Here's how the part is built. I have some questions about the finished solid (model axes, mm). Face numbers are marked on the shaded views. A direction names the side the tool comes from. Give positions to 0.01 mm unless a question says otherwise; leave off trailing zeros. Write each loop counter-clockwise with the first axis right and the second up, starting at its lowest first coordinate (ties: lowest second). Pieces come first, ordered by that corner, then holes. Notation, with made-up numbers: (65.25, -26.5) -> (94.25, -26.5) arc R35 ccw to (94.25, 6.5) -> close; hole circle Ø1 at (46, 18.5). An arc over 180 degrees is marked (long way). Use one line per item in the form item = value.
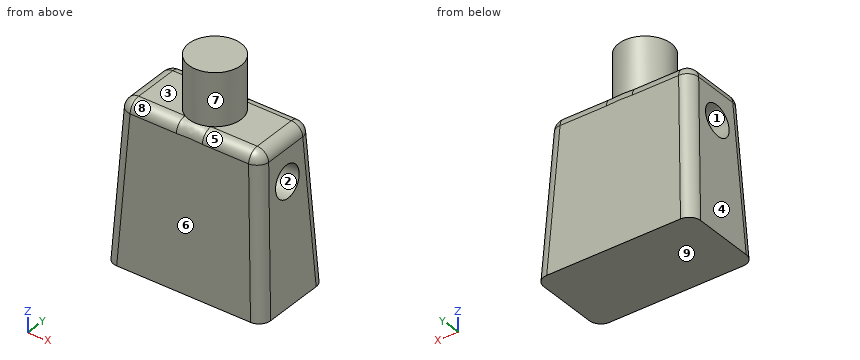
```python
from build123d import *

# Parameters (mm, degrees)
F0_W     = 15
F0_H     = 8
F1_DEPTH = 15
F1_TAPER = 3
F2_R     = 2.5
F3_DEPTH = 5
F4_R     = 1.1
F5_R     = 1.5
F6_DEPTH = 3
F7_R     = 1.5
F8_DEPTH = 3


with BuildPart() as f1:
    # F0 (on Top) → F1 (new body)
    with BuildSketch(Plane.XY):
        Rectangle(F0_W, F0_H)
    extrude(amount=F1_DEPTH, taper=F1_TAPER)

    # F2 (on face) → F3 (join)
    with BuildSketch(Plane.XY.offset(15)):
        Circle(F2_R)
    extrude(amount=F3_DEPTH)

    # F4
    f4_edges = [f1.edges().sort_by_distance(p)[0] for p in [
        (7.106942, 3.606942, 7.5),
        (-7.106942, 3.606942, 7.5),
        (0, 3.213883, 15),
        (-6.713883, 0, 15),
        (6.713883, 0, 15),
        (0, -3.213883, 15),
        (7.106942, -3.606942, 7.5),
        (-7.106942, -3.606942, 7.5),
    ]]
    fillet(f4_edges, radius=F4_R)

    # F5 (on face) → F6 (cut)
    with BuildSketch(Plane(origin=(-7.4794571076, 0, 0.3919817373), x_dir=(0, -1, 0), z_dir=(-0.9986295348, 0, 0.0523359562))):
        with Locations((0, 10.682696983)):
            Circle(F5_R)
    extrude(amount=-F6_DEPTH, mode=Mode.SUBTRACT)

    # F7 (on face) → F8 (cut)
    with BuildSketch(Plane(origin=(7.4794571076, 0, 0.3919817373), x_dir=(0, 1, 0), z_dir=(0.9986295348, 0, 0.0523359562))):
        with Locations((0, 10.682696983)):
            Circle(F7_R)
    extrude(amount=-F8_DEPTH, mode=Mode.SUBTRACT)


solid = f1.part
```
Q1. Which directions (+Z, -Z, +X, -X, +Y, -Y) give clear straight access to the entire face, cutting with the end or side of a thin tool? Please do the marked faces 5, 6, 7, 8 and 9.
Result set:
face_5 = +Z, +X, -Y
face_6 = +Z, +X, -X, -Y
face_7 = +Z
face_8 = +Z, -X, -Y
face_9 = -Z, +X, -X, +Y, -Y
Q2. I want a section at C-C, the plane z = 18.5. Write out the boundary of the cut face in (x, y), and give its area (3 significant figures).
Result set:
outline = circle Ø5 at (0, 0)
area = 19.6 mm2
Q3. I want a section at D-D, the plane y = -1. Write out the boundary of the cut face in (x, z), and give its area (3 significant figures).
Result set:
outline = (-7.5, 0) -> (7.5, 0) -> (6.98, 9.94) -> (3.98, 9.79) -> (3.87, 12.02) -> (6.86, 12.18) -> (6.77, 13.96) arc R1.1 ccw to (5.67, 15) -> (2.29, 15) -> (2.29, 20) -> (-2.29, 20) -> (-2.29, 15) -> (-5.67, 15) arc R1.1 ccw to (-6.77, 13.96) -> (-6.86, 12.18) -> (-3.87, 12.02) -> (-3.98, 9.79) -> (-6.98, 9.94) -> close
area = 222 mm2
Q4. If I drill on line 1 along Y through (x, z) = (2, 3); line 2 along Z through (x, y) = (-3, -1.25); line 3 along Y through (x, z) = (0, 16.5), over which ranges is the centre line in solid material (lowest first)? Write a range as from..to.
Result set:
line_1 = -3.84..3.84
line_2 = 0..15
line_3 = -2.5..2.5
Q5. I want a section at A-A, the plane x = -2.75. Write out the boundary of the cut face in (y, z).
Result set:
outline = (-4, 0) -> (4, 0) -> (3.27, 13.96) arc R1.1 ccw to (2.17, 15) -> (-2.17, 15) arc R1.1 ccw to (-3.27, 13.96) -> close
Q6. Will these pins go through, and if not, where does the flat tip stop? pin 1 Ø8 at (x, z) = (3.5, 17.5) entering from -Y; pin 2 Ø1 at (y, z) = (0.5, 11.5) entering from -X; pin 3 Ø5 at (x, z) = (-4, 5.5) entering from +Y.
Result set:
pin_1 = -3.29
pin_2 = -3.92
pin_3 = 3.84
Q7. I want a section at B-B, the plane y = 0. Write out the boundary of the cut face in (x, z).
Result set:
outline = (-7.5, 0) -> (7.5, 0) -> (7, 9.56) -> (4, 9.41) -> (3.85, 12.4) -> (6.84, 12.56) -> (6.77, 13.96) arc R1.1 ccw to (5.67, 15) -> (2.5, 15) -> (2.5, 20) -> (-2.5, 20) -> (-2.5, 15) -> (-5.67, 15) arc R1.1 ccw to (-6.77, 13.96) -> (-6.84, 12.56) -> (-3.85, 12.4) -> (-4, 9.41) -> (-7, 9.56) -> close
Q8. If we mould it in two halves opening along X, with no side actions, what happens to the marked faces 1, 2, 3 and 4? For each: +X half, -X half, draft (parallel to the pull), parting line (faces both ways), or undercut.
Result set:
face_1 = undercut
face_2 = undercut
face_3 = draft
face_4 = -X half
